Could you check a few things on this model? Use its own coordinates, in mm. A direction names the side the tool comes from. Round coordinates to 2 decimals unless told otherwise and drop trailing zeros. Loops run counter-clockwise (first coordinate to the right, second up) from the corner with the lowest first, then second, coordinate; pieces in that order, holes last. Notation, with made-up numbers: (21.5, 32.25) -> (58.5, 32.25) arc R16 cw to (58.5, 43.25) -> close; hole circle Ø10 at (35.25, 9.25). An arc over 180 degrees is marked (long way). One line per item, written item: value.
```python
from build123d import *

# Parameters (mm, degrees)
SKETCH_1_W                   = 150
SKETCH_1_H                   = 12
EXTRUDE_1_DEPTH              = 8
CUT_EXTRUDE_1_DEPTH          = 151.173233301
CUT_EXTRUDE_2_DEPTH          = 151.173233301
CUT_EXTRUDE_3_DEPTH          = 151.173233301
CUT_EXTRUDE_4_DEPTH          = 151.173233301
CUT_EXTRUDE_5_DEPTH          = 151.173233301
CUT_EXTRUDE_6_DEPTH          = 151.173233301
HOLE_WIZARD_M3_1_D           = 3.5
HOLE_WIZARD_M3_1_CBORE_D     = 5.9999
HOLE_WIZARD_M3_1_CBORE_DEPTH = 4.5
CHAMFER_1_SIZE               = 0.6
FILLET_1_R                   = 0.2


with BuildPart() as part:
    # 草图1 → 凸台-拉伸1 (new body)
    with BuildSketch(Plane(origin=(0, 4, 0), x_dir=(1, 0, 0), z_dir=(0, 1, 0))):
        Rectangle(SKETCH_1_W, SKETCH_1_H)
    extrude(amount=-EXTRUDE_1_DEPTH)

    # 草图2 → 切除-拉伸1 (cut, through all)
    with BuildSketch(Plane(origin=(75, 0, 0), x_dir=(0, 0, -1), z_dir=(1, 0, 0))):
        with BuildLine():
            Line((6, 1.51), (6, 2.01))
            Line((6, 2.01), (4.8, 2.01))
            ThreePointArc((4.8, 2.01), (4.55, 1.76), (4.8, 1.51))
            Line((4.8, 1.51), (6, 1.51))
        make_face()
    extrude(amount=-CUT_EXTRUDE_1_DEPTH, mode=Mode.SUBTRACT)

    # 草图3 → 切除-拉伸2 (cut, through all)
    with BuildSketch(Plane(origin=(75, 0, 0), x_dir=(0, 0, -1), z_dir=(1, 0, 0))):
        with BuildLine():
            Line((6, 2.01), (6, 3.111111))
            ThreePointArc((6, 3.111111), (5.367595703, 2.693428684), (5.04, 2.01))
            Line((5.04, 2.01), (6, 2.01))
        make_face()
    extrude(amount=-CUT_EXTRUDE_2_DEPTH, mode=Mode.SUBTRACT)

    # 草图4 → 切除-拉伸3 (cut, through all)
    with BuildSketch(Plane(origin=(75, 0, 0), x_dir=(0, 0, -1), z_dir=(1, 0, 0))):
        with BuildLine():
            Line((6, 1.51), (5.04, 1.51))
            ThreePointArc((5.04, 1.51), (5.367595703, 0.826571316), (6, 0.408889))
            Line((6, 0.408889), (6, 1.51))
        make_face()
    extrude(amount=-CUT_EXTRUDE_3_DEPTH, mode=Mode.SUBTRACT)

    # 草图5 → 切除-拉伸4 (cut, through all)
    with BuildSketch(Plane(origin=(75, 0, 0), x_dir=(0, 0, -1), z_dir=(1, 0, 0))):
        with BuildLine():
            Line((-6, 2.01), (-6, 1.51))
            Line((-6, 1.51), (-4.8, 1.51))
            ThreePointArc((-4.8, 1.51), (-4.55, 1.76), (-4.8, 2.01))
            Line((-4.8, 2.01), (-6, 2.01))
        make_face()
    extrude(amount=-CUT_EXTRUDE_4_DEPTH, mode=Mode.SUBTRACT)

    # 草图6 → 切除-拉伸5 (cut, through all)
    with BuildSketch(Plane(origin=(75, 0, 0), x_dir=(0, 0, -1), z_dir=(1, 0, 0))):
        with BuildLine():
            Line((-6, 1.51), (-6, 0.408889))
            ThreePointArc((-6, 0.408889), (-5.367595703, 0.826571316), (-5.04, 1.51))
            Line((-5.04, 1.51), (-6, 1.51))
        make_face()
    extrude(amount=-CUT_EXTRUDE_5_DEPTH, mode=Mode.SUBTRACT)

    # 草图7 → 切除-拉伸6 (cut, through all)
    with BuildSketch(Plane(origin=(75, 0, 0), x_dir=(0, 0, -1), z_dir=(1, 0, 0))):
        with BuildLine():
            Line((-6, 2.01), (-5.04, 2.01))
            ThreePointArc((-5.04, 2.01), (-5.367595703, 2.693428684), (-6, 3.111111))
            Line((-6, 3.111111), (-6, 2.01))
        make_face()
    extrude(amount=-CUT_EXTRUDE_6_DEPTH, mode=Mode.SUBTRACT)

    # M3 六角头机械螺钉的柱形沉头孔1 (through all)
    with Locations(Plane(origin=(0, 4, 0), x_dir=(1, 0, 0), z_dir=(0, 1, 0))):
        with Locations((-62.5, 0), (-37.5, 0), (-12.5, 0), (12.5, 0), (37.5, 0), (62.5, 0)):
            CounterBoreHole(HOLE_WIZARD_M3_1_D / 2, HOLE_WIZARD_M3_1_CBORE_D / 2, HOLE_WIZARD_M3_1_CBORE_DEPTH)

    # 倒角1
    chamfer_1_edges = [part.edges().sort_by_distance(p)[0] for p in [
        (0, -4, -6),
        (0, -4, 6),
    ]]
    chamfer(chamfer_1_edges, length=CHAMFER_1_SIZE)

    # 圆角1
    fillet_1_edges = [part.edges().sort_by_distance(p)[0] for p in [
        (0, 2.01, -5.04),
        (0, 3.111111, -6),
        (0, 0.408889, -6),
        (0, 1.51, -5.04),
        (0, 4, -6),
        (0, 4, 6),
        (0, 1.51, 5.04),
        (0, 0.408889, 6),
        (0, 3.111111, 6),
        (0, 2.01, 5.04),
    ]]
    fillet(fillet_1_edges, radius=FILLET_1_R)


solid = part.part
```
(1) On a 3-axis mill with a long thin cutter (end or side, diameter ignored), from which of +Z, -Z, +X, -X, +Y, -Y can I reach the whole of each face in a straight line? I mean faces 5 (the face through (-13, -0.5, 2)), 6 (the face through (-1, -4, 0)). Say none if no direction works.
Results below:
face 5: +Y
face 6: +Z, -Z, +X, -X, -Y
(2) For pin 1 Ø1.8 at (x, z) = (-62.5, -1.5) entering from +Y; pin 2 Ø1 at (x, y) = (12, 2.5) entering from +Z, each with a flat end and sliding along its axis, tell me the tip position at first contact or that it passes through.
Results below:
pin 1: stops at y = -0.5
pin 2: stops at z = 5.75
(3) Imagine slicing it at A-A on x = -52.5. Write out the boundary of the cut face in (y, z).
Results below:
outline: (-4, -5.4) -> (-3.4, -6) -> (0.27, -6) arc R0.2 ccw to (0.45, -5.88) arc R1.42 cw to (1.37, -5.07) arc R0.2 ccw to (1.51, -4.88) -> (1.51, -4.8) arc R0.25 cw to (2.01, -4.8) -> (2.01, -4.88) arc R0.2 ccw to (2.15, -5.07) arc R1.42 cw to (3.07, -5.88) arc R0.2 ccw to (3.25, -6) -> (3.8, -6) arc R0.2 ccw to (4, -5.8) -> (4, 5.8) arc R0.2 ccw to (3.8, 6) -> (3.25, 6) arc R0.2 ccw to (3.07, 5.88) arc R1.42 cw to (2.15, 5.07) arc R0.2 ccw to (2.01, 4.88) -> (2.01, 4.8) arc R0.25 cw to (1.51, 4.8) -> (1.51, 4.88) arc R0.2 ccw to (1.37, 5.07) arc R1.42 cw to (0.45, 5.88) arc R0.2 ccw to (0.27, 6) -> (-3.4, 6) -> (-4, 5.4) -> close
(4) We'd pull the mould along X, two halves only. Please class faces 1 (the face through (-64.169, -2.274, -0.526)), 2 (the face through (-1, -2, -6)), 3 (the face through (-60.5, -0.5, 0)), 4 (the face through (75, 0, 0)): +X half, -X half, draft (parallel to the pull), parting line (faces both ways), or undercut.
Results below:
face 1: undercut
face 2: draft
face 3: undercut
face 4: +X half
(5) Please list where these lines run through material, in increasing order: L1, parallel to Y at x = -26, z = 4.75; L2, parallel to Z at x = 62.5, y = -1.5; L3, parallel to Z at x = -12.5, y = 2.15.
Results below:
L1: y = -4 to 1.52, 2 to 4
L2: z = -6 to -1.75, 1.75 to 6
L3: z = -5.07 to -3, 3 to 5.07
